Input: part model. Units: mm. Frame: model coordinates. A direction names the side the tool comes from. Give positions to 0.01 mm unless a question says otherwise; leave off trailing zeros. Loops run counter-clockwise (first coordinate to the right, second up) from the corner with the lowest first, then second, coordinate; pieces in that order, holes last. Notation, with made-up numbers: (69, -15) - (123, -15) arc R23 cw to (123, 4) - close; hole circle Ø4 at (37, -13). An arc over 180 degrees is marked (long way). Answer as a JSON object with one key per item and string values. Group by question number.
(1) Access query for faces 5 (the flat face through (4, 4, 2)), 6 (the flat face through (-5, 7, -3)). Directions: +Z, -Z, +X, -X, +Y, -Y. A direction counts if a zero-diameter tool reaches every point of the face in a straight line with its end or side. Return the directions, or none.
(2) Section query B-B (x = 0). Return loops of the section in (y, z), plus the area to 3 significant figures.
(3) Section query D-D (z = -3.5). Return loops of the section in (x, y), plus the area to 3 significant figures.
(4) Material intervals for L1, parallel to Y at x = 0, z = 1.5; L2, parallel to Y at x = -1.75, z = 1; L3, parallel to X at y = -2.5, z = 1.75, sorted ascending.
(5) Pin query (flat end, axial travel): P1, Ø1.5, axis at y = 4, z = -1.5, coming from the +X side; P2, Ø3, axis at y = 4.5, z = 0.5, coming from the -X side; P3, Ø1, axis at y = -3, z = -1, coming from the -X side. Return the tip coordinate at first contact, or that it passes through.
(6) Section query C-C (z = -1). Return loops of the section in (x, y).
(7) Section query A-A (y = 0). Return loops of the section in (x, z).
(8) Mould query, pull axis X, two halves, no side actions, for faces 1 (the flat face through (7.329, -4.306, -0.465)), 2 (the flat face through (-7.394, -4.194, -0.465)), 3 (the flat face through (0, -8.5, 0)), 4 (the cylindrical face through (-1.73, 7.81, -3.34)). Classes: +X half, -X half, draft (parallel to the pull), parting line (faces both ways), or undercut.
```python
from build123d import *

# Parameters (mm, degrees)
ESQUISSE2_R             = 11.85785331
ENL_V_MAT_EXTRU_1_DEPTH = 10


with BuildPart() as part:
    # Esquisse1 → R_volution1 (revolve)
    with BuildSketch(Plane(origin=(0, 0, 0), x_dir=(0, 0, -1), z_dir=(1, 0, 0)), mode=Mode.PRIVATE) as r_volution1_sk:
        with BuildLine():
            Line((-1.6, 4.5), (4, 4.5))
            Line((4, 4.5), (4, 8))
            Line((4, 8), (3, 8))
            Line((3, 8), (2.7, 8))
            Line((2.7, 8), (2.7, 8.4))
            Line((2.7, 8.4), (3, 8.4))
            Line((3, 8.4), (3, 9.774245233))
            ThreePointArc((3, 9.774245233), (2.898746035, 9.889790175), (2.791709623, 10))
            Line((2.791709623, 10), (-1.191709623, 10))
            ThreePointArc((-1.191709623, 10), (-1.691931822, 9.355470088), (-2, 8.6))
            Line((-2, 8.6), (-2, 4.9))
            Line((-2, 4.9), (-1.6, 4.5))
        make_face()
    revolve(r_volution1_sk.sketch.rotate(Axis((0, 0, 15.19936), (0, 0, -1)), 90), axis=Axis((0, 0, 15.19936), (0, 0, -1)))

    # Esquisse2 → Enl_v. mat.-Extru.1 (cut)
    with BuildSketch(Plane.XY.offset(2)):
        Circle(ESQUISSE2_R)
        with BuildLine():
            Line((-5.051814855, 8.25), (-9.670617009, 0.25))
            ThreePointArc((-9.670617009, 0.25), (-9.737604307, 0), (-9.670617009, -0.25))
            Line((-9.670617009, -0.25), (-5.051814855, -8.25))
            ThreePointArc((-5.051814855, -8.25), (-4.868802154, -8.433012702), (-4.618802154, -8.5))
            Line((-4.618802154, -8.5), (4.618802154, -8.5))
            ThreePointArc((4.618802154, -8.5), (4.868802154, -8.433012702), (5.051814855, -8.25))
            Line((5.051814855, -8.25), (9.670617009, -0.25))
            ThreePointArc((9.670617009, -0.25), (9.737604307, 0), (9.670617009, 0.25))
            Line((9.670617009, 0.25), (5.051814855, 8.25))
            ThreePointArc((5.051814855, 8.25), (4.868802154, 8.433012702), (4.618802154, 8.5))
            Line((4.618802154, 8.5), (-4.618802154, 8.5))
            ThreePointArc((-4.618802154, 8.5), (-4.868802154, 8.433012702), (-5.051814855, 8.25))
        make_face(mode=Mode.SUBTRACT)
    extrude(amount=-ENL_V_MAT_EXTRU_1_DEPTH, mode=Mode.SUBTRACT)


solid = part.part
```
Recorded:
{
 "1": {"face 5": "+Z, +X, -X, +Y, -Y", "face 6": "-Z"},
 "2": {"outline": "(-8.5, -3) - (-8.4, -3) - (-8.4, -2.7) - (-8, -2.7) - (-8, -4) - (-4.5, -4) - (-4.5, 1.6) - (-4.9, 2) - (-8.5, 2) - close; (4.5, -4) - (8, -4) - (8, -2.7) - (8.4, -2.7) - (8.4, -3) - (8.5, -3) - (8.5, 2) - (4.9, 2) - (4.5, 1.6) - close", "area": "46.6 mm^2"},
 "3": {"outline": "circle Ø16 at (0, 0); hole circle Ø9 at (0, 0)", "area": "137 mm^2"},
 "4": {"L1": "y = -8.5 to -4.5, 4.5 to 8.5", "L2": "y = -8.5 to -4.15, 4.15 to 8.5", "L3": "x = -8.37 to -3.92, 3.92 to 8.37"},
 "5": {"P1": "stops at x = 7.94", "P2": "stops at x = -8.08", "P3": "stops at x = -8.37"},
 "6": {"outline": "(-9.67, -0.25) - (-5.05, -8.25) arc R0.5 ccw to (-4.62, -8.5) - (4.62, -8.5) arc R0.5 ccw to (5.05, -8.25) - (9.67, -0.25) arc R0.5 ccw to (9.67, 0.25) - (5.05, 8.25) arc R0.5 ccw to (4.62, 8.5) - (-4.62, 8.5) arc R0.5 ccw to (-5.05, 8.25) - (-9.67, 0.25) arc R0.5 ccw to start; hole circle Ø9 at (0, 0)"},
 "7": {"outline": "(-9.74, -3) - (-8.4, -3) - (-8.4, -2.7) - (-8, -2.7) - (-8, -4) - (-4.5, -4) - (-4.5, 1.6) - (-4.9, 2) - (-8.6, 2) arc R3 ccw to (-9.74, 1.43) - close; (4.5, -4) - (8, -4) - (8, -2.7) - (8.4, -2.7) - (8.4, -3) - (9.74, -3) - (9.74, 1.43) arc R3 ccw to (8.6, 2) - (4.9, 2) - (4.5, 1.6) - close"},
 "8": {"face 1": "+X half", "face 2": "-X half", "face 3": "draft", "face 4": "undercut"}
}
